The drawing under review shows one solid part. Ordinate dimensions are in mm from its lowest x, y, z. A direction names the side the tool comes from. Coordinates: 2 decimals unless noted, no trailing zeros. Write each loop counter-clockwise with the first axis right and the second up, starting at its lowest first coordinate (ties: lowest second). Pieces come first, ordered by that corner, then holes. Notation, with made-up numbers: (76.5, 21.5) - (104.5, 21.5) arc R9 ccw to (104.5, 28.5) - close; hole circle Ø10 at (-31.75, 65.5). An arc over 180 degrees is marked (long way). Put each result on its own line as item: value. Start each with the question number.
Item 1: Consider section B-B on x = 22.5. Give the boundary of the cut face in (y, z).
Item 2: Consider section A-A on z = 5. Give the boundary of the cut face in (x, y).
Item 3: Mouldability with a two-part tool opening along X and no side actions: class the marked faces 4 and 5 as pulls with the +X half, pulls with the -X half, needs draft (parallel to the pull), parting line crosses it, or undercut.
Item 4: To check wall thickness, follow L1, parallel to Y at x = 17.5, z = 14; L2, parallel to X at y = 20.5, z = 6.25; L3, parallel to X at y = 16, z = 2. State the ranges of each line that lie inside material, in increasing order. Write a range as [from, to].
Item 5: Consider section D-D on y = 12.5. Give the boundary of the cut face in (x, z).
Item 6: For pin 1 (10 mm diameter, centred on x = 87, z = 7.5, fed in from -Y); pin 2 (1 mm diameter, centred on x = 79, z = 4, fed in from +Y); pin 3 (1.5 mm diameter, centred on y = 15, z = 11.5, fed in from -X), all flat-tipped, find the tip position at first contact; note any pin that passes through.
Item 7: Machinability: for the marked faces 1, 2 and 3, which of the approach directions +Z, -Z, +X, -X, +Y, -Y give a long, thin tool a straight path to every point of the face, cutting with its end or side? Answer none if there is none.
Item 8: Consider section C-C on y = 29.5. Give the boundary of the cut face in (x, z).
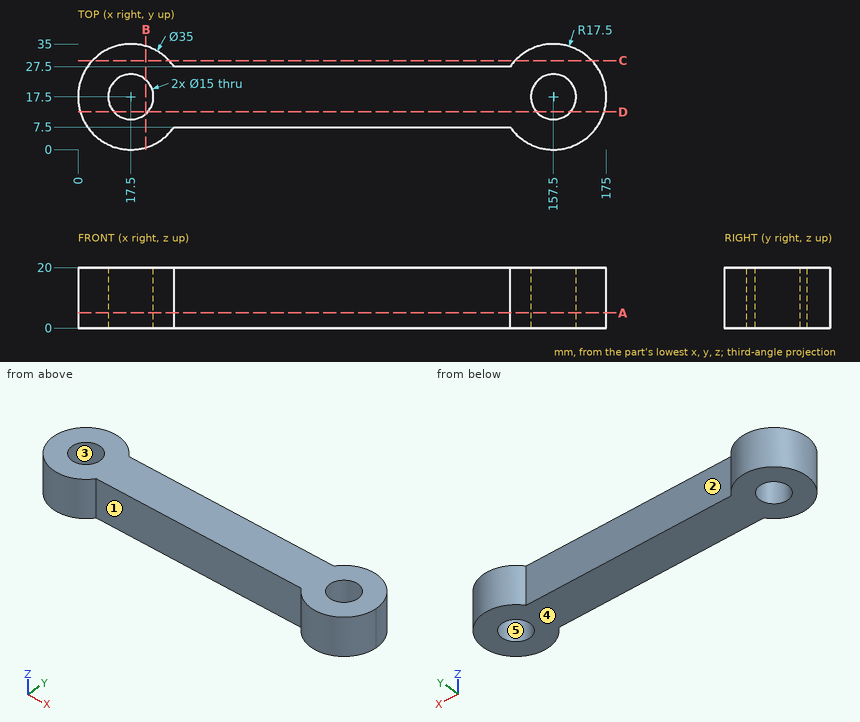
Report:
1. outline: (0.73, 0) - (11.91, 0) - (11.91, 20) - (0.73, 20) - close; (23.09, 0) - (34.27, 0) - (34.27, 20) - (23.09, 20) - close
2. outline: (31.86, 7.5) - (143.14, 7.5) arc R17.5 ccw (long way) to (143.14, 27.5) - (31.86, 27.5) arc R17.5 ccw (long way) to start; hole circle Ø15 at (17.5, 17.5); hole circle Ø15 at (157.5, 17.5)
3. face 4: needs draft
3. face 5: undercut
4. L1: [0, 10], [25, 35]
4. L2: [0.26, 10.63], [24.37, 150.63], [164.37, 174.74]
4. L3: [0.06, 10.15], [24.85, 150.15], [164.85, 174.94]
5. outline: (0.73, 0) - (11.91, 0) - (11.91, 20) - (0.73, 20) - close; (23.09, 0) - (151.91, 0) - (151.91, 20) - (23.09, 20) - close; (163.09, 0) - (174.27, 0) - (174.27, 20) - (163.09, 20) - close
6. pin 1: y = 7.5
6. pin 2: y = 27.5
6. pin 3: x = 0.09
7. face 1: +Z, -Z, -Y
7. face 2: +Z, -Z, +Y
7. face 3: +Z, -Z
8. outline: (4.76, 0) - (30.24, 0) - (30.24, 20) - (4.76, 20) - close; (144.76, 0) - (170.24, 0) - (170.24, 20) - (144.76, 20) - close
